Autodesk Inventor part; units mm, degrees
ref_plane "YZ Plane" through (0, 0, 0) normal (1, 0, 0) x (0, 1, 0)
ref_plane "XZ Plane" through (0, 0, 0) normal (0, 1, 0) x (-1, 0, 0)
ref_plane "XY Plane" through (0, 0, 0) normal (0, 0, 1) x (1, 0, 0)
sketch "Sketch1" plane through (0, 0, 0) normal (0, 1, 0) x (-1, 0, 0)
  line L0 (40.8683, 149.0264) -> (9.5242, 149.0264)
  line L1 (9.5242, -50.9736) -> (40.8683, -50.9736)
  line L2 (40.8683, -50.9736) -> (40.8683, 149.0264)
  line L3 (9.5242, 118.5264) -> (2.5242, 118.5264)
  line L4 (2.5242, 118.5264) -> (2.5242, 79.5264)
  line L5 (2.5242, 79.5264) -> (9.5242, 79.5264)
  line L6 (9.5242, 18.5264) -> (2.5242, 18.5264)
  line L7 (2.5242, 18.5264) -> (2.5242, -20.4736)
  line L8 (2.5242, -20.4736) -> (9.5242, -20.4736)
  line L9 (9.5242, 149.0264) -> (9.5242, 118.5264)
  line L10 (9.5242, 79.5264) -> (9.5242, 18.5264)
  line L11 (9.5242, -20.4736) -> (9.5242, -50.9736)
  point P0 (0, 0)
  dimension "d1" = 200
  dimension "d2" = 30.5
  dimension "d3" = 30.5
  dimension "d4" = 61
  dimension "d5" = 39
  dimension "d6" = 7
extrude "Extrusion1" add sketch "Sketch1" along normal blind 3
properties part number "track_guides_3mm"
Read the model definition and answer for the solid it produces. Units are mm, in the model's axes. Round coordinates to 2 decimals unless told otherwise and drop trailing zeros. Loops run counter-clockwise (first coordinate to the right, second up) from the corner with the lowest first, then second, coordinate; pieces in that order, holes last. Notation, with made-up numbers: (13.25, 82.25) - (61.25, 82.25) arc R15 ccw to (61.25, 110.25) - close; hole circle Ø6 at (73.25, 28). An arc over 180 degrees is marked (long way). One line per question, with ' | ' between items. Start each with the question number.
Q1. Find the intervals of material crossed by L1, parallel to Z at x = -4.5, y = 1.7; L2, parallel to X at y = 1.25, z = 76.5, in increasing order.
Q2. Section A-A on y = 1.9 is taken. Give the vertices of the cut face in (x, z).
Q3. Flat-ended cylindrical pins translate along their axes: pin 1 (1.5 mm diameter, centred on x = -7, y = 1, fed in from +Z); pin 2 (1.5 mm diameter, centred on x = -6, y = 1.5, fed in from -Z); pin 3 (0.9 mm diameter, centred on y = 2, z = 55, fed in from +X). Find the tip coordinate at first contact, or state that the pin passes through.
Q4. Section B-B on z = -23 is taken. Give the vertices of the cut face in (x, y), plus the area to 3 significant figures.
Established:
1) L1: -20.47 to 18.53, 79.53 to 118.53 | L2: -40.87 to -9.52
2) outline: (-40.87, -50.97) - (-9.52, -50.97) - (-9.52, -20.47) - (-2.52, -20.47) - (-2.52, 18.53) - (-9.52, 18.53) - (-9.52, 79.53) - (-2.52, 79.53) - (-2.52, 118.53) - (-9.52, 118.53) - (-9.52, 149.03) - (-40.87, 149.03) - close
3) pin 1: z = 118.53 | pin 2: z = -20.47 | pin 3: x = -9.52
4) outline: (-40.87, 0) - (-9.52, 0) - (-9.52, 3) - (-40.87, 3) - close | area: 94.0 mm²
